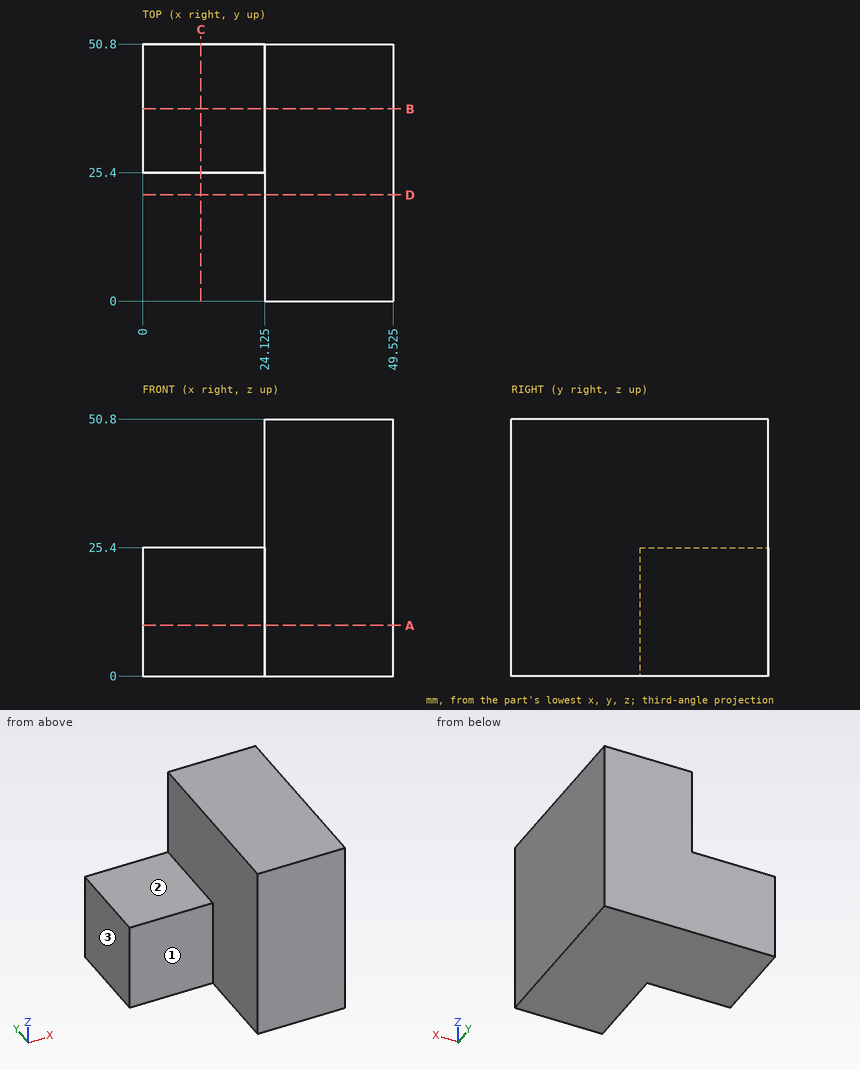
Job drawing, mm, ordinate dimensions from the low corner. One solid piece. A direction names the side the tool comes from. Coordinates: 2 decimals unless noted, no trailing zeros. Order: outer loops, then holes, each group sorted by start corner. A loop starts at its lowest first (then second) coordinate and runs counter-clockwise, first axis right, second up. Notation, with made-up numbers: (-13, 8) -> (6, 8) arc R19 ccw to (6, 19) -> close; hole circle Ø10 at (59.5, 74.5). An arc over 180 degrees is marked (long way). Put each result on its own line as item: value. Start each with the question number.
(1) Which spindle directions (+Z, -Z, +X, -X, +Y, -Y) get a long thin tool onto all of the face, cutting with end or side? Do the marked faces 1, 2 and 3. Say none if no direction does.
(2) Band-saw the part on B-B (y = 38). Give the cut face in (x, z) (1 decimal).
(3) Band-saw the part on D-D (y = 21). Give the cut face in (x, z) (1 decimal).
(4) Pin check, flat tips, straight feed: pin 1 Ø1.5 at (y, z) = (12.5, 36.5) entering from -X (1 decimal); pin 2 Ø3 at (x, z) = (10, 5.5) entering from -Y; pin 3 Ø7 at (x, y) = (6.5, 42.5) entering from +Z. Stop position of each tip, or through.
(5) Band-saw the part on C-C (x = 11.5). Give the cut face in (y, z), then the cut area to 3 significant figures.
(6) Band-saw the part on A-A (z = 10). Give the cut face in (x, y) (1 decimal).
(7) Probe line 1 along Y through (x, z) = (14.5, 5.5); line 2 along X through (y, z) = (23.5, 24) (1 decimal); line 3 along Z through (x, y) = (15, 35). List the from-to ranges inside material, lowest first. Write a range as [from, to].
Determined:
1. face 1: +Z, -Z, -X, -Y
1. face 2: +Z, -X, +Y, -Y
1. face 3: +Z, -Z, -X, +Y, -Y
2. outline: (0, 0) -> (49.5, 0) -> (49.5, 50.8) -> (24.1, 50.8) -> (24.1, 25.4) -> (0, 25.4) -> close
3. outline: (24.1, 0) -> (49.5, 0) -> (49.5, 50.8) -> (24.1, 50.8) -> close
4. pin 1: stops at x = 24.1
4. pin 2: stops at y = 25.4
4. pin 3: stops at z = 25.4
5. outline: (25.4, 0) -> (50.8, 0) -> (50.8, 25.4) -> (25.4, 25.4) -> close
5. area: 645 mm²
6. outline: (0, 25.4) -> (24.1, 25.4) -> (24.1, 0) -> (49.5, 0) -> (49.5, 50.8) -> (0, 50.8) -> close
7. line 1: y = [25.4, 50.8]
7. line 2: x = [24.1, 49.5]
7. line 3: z = [0, 25.4]
